from build123d import *

# Parameters (mm, degrees)
BASIS_DEKSEL_DEPTH = 3
UITSPARING_DEPTH   = 157.456721252


with BuildPart() as part:
    # basis_deksel_schets → basis_deksel (new body)
    with BuildSketch(Plane(origin=(0, 0, 0), x_dir=(1, 0, 0), z_dir=(0, 1, 0))):
        with BuildLine():
            Line((-98, 23.925), (0, 121.925))
            Line((0, 121.925), (98, 23.925))
            Line((98, 23.925), (98, 23.225))
            ThreePointArc((98, 23.225), (84.190084733, -10.115084733), (50.85, -23.925))
            Line((50.85, -23.925), (-50.85, -23.925))
            ThreePointArc((-50.85, -23.925), (-84.190084733, -10.115084733), (-98, 23.225))
            Line((-98, 23.225), (-98, 23.925))
        make_face()
    extrude(amount=BASIS_DEKSEL_DEPTH)

    # uitsparing_schets → uitsparing (cut, through all)
    with BuildSketch(Plane(origin=(0, 3, 0), x_dir=(1, 0, 0), z_dir=(0, 1, 0))):
        with BuildLine():
            Line((-15, -23.925), (15, -23.925))
            ThreePointArc((15, -23.925), (0, -8.925), (-15, -23.925))
        make_face()
    extrude(amount=-UITSPARING_DEPTH, mode=Mode.SUBTRACT)


solid = part.part
Design review of the part built by this model. Coordinates are the model's own, in mm. Give positions to 0.01 mm unless a question says otherwise; leave off trailing zeros. Loops run counter-clockwise (first coordinate to the right, second up) from the corner with the lowest first, then second, coordinate; pieces in that order, holes last. Notation, with made-up numbers: M 0.25,-31.5 L 13.25,-31.5 A20 ccw 13.25,-1.5 Z; hole C 10.5,32 d4. An arc over 180 degrees is marked long. Answer as a JSON object with one key per item and string values.
Item 1: We need section B-B (x = -67). State the section outline as (y, z) points (3 decimals).
Output values:
{"outline": "M 0,-54.925 L 3,-54.925 L 3,21.073 L 0,21.073 Z"}
Item 2: Wall thickness on line 1 along X through (y, z) = (2.7, 16.5); line 2 along Z through (x, y) = (-74, 1.25) (3 decimals); line 3 along X through (y, z) = (2.25, 6): over which ranges is each line inside the solid? List them lowest first.
Output values:
{"line 1": "x = -76.25 to -13.03, 13.03 to 76.25", "line 2": "z = -47.925 to 17.851", "line 3": "x = -87.85 to 87.85"}
Item 3: We need section C-C (z = -99). State the section outline as (x, y) points (3 decimals), and give its area (3 significant figures).
Output values:
{"outline": "M -22.925,0 L 22.925,0 L 22.925,3 L -22.925,3 Z", "area": "138 mm2"}
Item 4: We need section A-A (y = 1.6). State the section outline as (x, z) points (3 decimals).
Output values:
{"outline": "M -98,-23.925 L 0,-121.925 L 98,-23.925 L 98,-23.225 A47.15 ccw 50.85,23.925 L 15,23.925 A15 cw -15,23.925 L -50.85,23.925 A47.15 ccw -98,-23.225 Z"}
Item 5: For P1, Ø1.5, axis at y = 1.5, z = -2.5, coming from the +X side; P2, Ø1, axis at y = 1.5, z = -14.5, coming from the -X side, all flat-tipped, find the tip position at first contact; note any pin that passes through.
Output values:
{"P1": "stops at x = 93.56", "P2": "stops at x = -97.28"}
